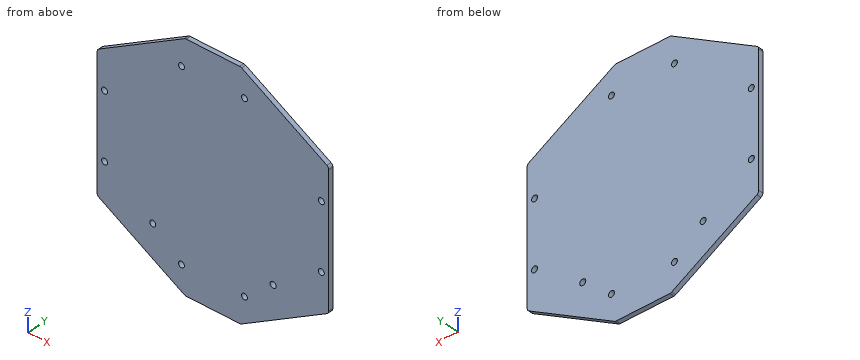
```python
from build123d import *

# Parameters (mm, degrees)
BOSS_EXTRUDE1_DEPTH     = 2.5
SKETCH3_R               = 1.6
CUT_EXTRUDE1_DEPTH      = 10
SKETCH5_R               = 1.625
CUT_EXTRUDE2_DEPTH      = 10
CUT_EXTRUDE3_DEPTH      = 90.139403932
CUT_EXTRUDE3_DEPTH_BACK = 90.139403932
SKETCH6_R               = 1.625
FILLET1_R               = 2


with BuildPart() as part:
    # Sketch1 → Boss-Extrude1 (new body)
    with BuildSketch(Plane(origin=(0, 0, 0), x_dir=(1, 0, 0), z_dir=(0, 1, 0))):
        Polygon((-15, 63.508529611), (15, 63.508529611), (62.5, 36.084391824), (62.5, -36.084391824), (15, -63.508529611), (-15, -63.508529611), (-62.5, -36.084391824), (-62.5, 36.084391824), align=None)
    extrude(amount=BOSS_EXTRUDE1_DEPTH)

    # Sketch3 → Cut-Extrude1 (cut)
    with BuildSketch(Plane.XZ):
        with Locations(Location((17, 49, 0), (0, 0, 270))):
            Circle(SKETCH3_R)
        with Locations(Location((-17, 49, 0), (0, 0, 270))):
            Circle(SKETCH3_R)
        with Locations(Location((17, -49, 0), (0, 0, 90))):
            Circle(SKETCH3_R)
        with Locations(Location((-17, -49, 0), (0, 0, 90))):
            Circle(SKETCH3_R)
    extrude(amount=-CUT_EXTRUDE1_DEPTH, mode=Mode.SUBTRACT)

    # Sketch5 → Cut-Extrude2 (cut)
    with BuildSketch(Plane(origin=(0, 2.5, 0), x_dir=(1, 0, 0), z_dir=(0, 1, 0))):
        with Locations(Location((-32.5, 36, 0), (0, 0, 270))):
            Circle(SKETCH5_R)
        with Locations(Location((32.5, 36, 0), (0, 0, 270))):
            Circle(SKETCH5_R)
    extrude(amount=-CUT_EXTRUDE2_DEPTH, mode=Mode.SUBTRACT)

    # Sketch6 → Cut-Extrude3 (cut, two sides: drawn at the far end of the back side and taken through both)
    with BuildSketch(Plane(origin=(0, 2.5, 0), x_dir=(1, 0, 0), z_dir=(0, 1, 0)).offset(-CUT_EXTRUDE3_DEPTH_BACK)):
        with Locations(Location((-58.5, 17.5, 0), (0, 0, 270))):
            Circle(SKETCH6_R)
        with Locations(Location((-58.5, -17.5, 0), (0, 0, 270))):
            Circle(SKETCH6_R)
        with Locations(Location((58.5, -17.5, 0), (0, 0, 270))):
            Circle(SKETCH6_R)
        with Locations(Location((58.5, 17.5, 0), (0, 0, 270))):
            Circle(SKETCH6_R)
    extrude(amount=CUT_EXTRUDE3_DEPTH + CUT_EXTRUDE3_DEPTH_BACK, mode=Mode.SUBTRACT)

    # Fillet1
    fillet1_edges = [part.edges().sort_by_distance(p)[0] for p in [
        (-15, 1.25, -63.508529611),
        (15, 1.25, -63.508529611),
        (62.5, 1.25, -36.084391824),
        (62.5, 1.25, 36.084391824),
        (15, 1.25, 63.508529611),
        (-15, 1.25, 63.508529611),
        (-62.5, 1.25, 36.084391824),
        (-62.5, 1.25, -36.084391824),
    ]]
    fillet(fillet1_edges, radius=FILLET1_R)


solid = part.part
```
Part model, mm, in its own coordinate system. Round coordinates to 2 decimals unless told otherwise and drop trailing zeros. Write each loop counter-clockwise with the first axis right and the second up, starting at its lowest first coordinate (ties: lowest second). Pieces come first, ordered by that corner, then holes. Notation, with made-up numbers: M -1,13.5 L 56,13.5 A13 ccw 56,25.5 Z; hole C -7,-17.5 d10. An arc over 180 degrees is marked long. Answer as CSV lines item,"result". Start each with the question number.
1) Drill centre lines: L1, parallel to X at y = 0.9, z = 17.5 (3 decimals); L2, parallel to X at y = 0.8, z = -35; L3, parallel to Z at x = -58.5, y = 0.95 (3 decimals). Where is each one in solid material? Low to high.
2) Band-saw the part on A-A (y = 0.8). Count the separate pieces of the cut face and the enclosed holes in it, then the cut area to 3 significant figures.
3) Band-saw the part on D-D (x = 32.5). List the corners of the cut face in (y, z) (3 decimals), then the cut area to 3 significant figures.
4) Band-saw the part on B-B (z = 17.5). List the corners of the cut face in (x, y) (3 decimals).
5) Band-saw the part on C-C (x = 17). List the corners of the cut face in (y, z), then the cut area to 3 significant figures.
Worked out:
1,L1,"-62.5 to -60.125, -56.875 to 56.875, 60.125 to 62.5"
1,L2,"-62.5 to -33.78, -31.22 to 31.22, 33.78 to 62.5"
1,L3,"-38.394 to -19.125, -15.875 to 15.875, 19.125 to 38.394"
2,separate pieces,"1"
2,enclosed holes,"10"
2,area,"13,200 mm²"
3,outline,"M 0,-53.405 L 2.5,-53.405 L 2.5,-37.625 L 0,-37.625 Z; M 0,-34.375 L 2.5,-34.375 L 2.5,53.405 L 0,53.405 Z"
3,area,"259 mm²"
4,outline,"M -62.5,0 L -60.125,0 L -60.125,2.5 L -62.5,2.5 Z; M -56.875,0 L 56.875,0 L 56.875,2.5 L -56.875,2.5 Z; M 60.125,0 L 62.5,0 L 62.5,2.5 L 60.125,2.5 Z"
5,outline,"M 0,-62.35 L 2.5,-62.35 L 2.5,-50.6 L 0,-50.6 Z; M 0,-47.4 L 2.5,-47.4 L 2.5,47.4 L 0,47.4 Z; M 0,50.6 L 2.5,50.6 L 2.5,62.35 L 0,62.35 Z"
5,area,"296 mm²"
